Source: CAD feature listing. Evaluate the final solid. Frame: model axes, mm. Face numbers are marked on the shaded views. A direction names the side the tool comes from. Give positions to 0.01 mm unless a question says otherwise; leave off trailing zeros. Write each loop counter-clockwise with the first axis right and the second up, starting at its lowest first coordinate (ties: lowest second). Pieces come first, ordered by that corner, then holes. Notation, with made-up numbers: (8, 22) -> (55, 22) arc R21 cw to (55, 43) -> close; hole circle Ø11 at (77, -1). An arc over 180 degrees is marked (long way). Answer as a JSON object with one key per item and string values. Group by question number.
Item 1: Pull-direction query (Z, two-part tool) for the marked faces 1, 2 and 3; classes: pulls with the +Z half, pulls with the -Z half, needs draft (parallel to the pull), parting line crosses it, or undercut.
Item 2: First-contact query: pin 1 Ø7.5 at (x, y) = (92, 1) entering from -Z; pin 2 Ø7 at (x, z) = (90.5, -31) entering from +Y; pin 3 Ø4.5 at (x, y) = (-1, -5.5) entering from +Z; pin 4 Ø4 at (x, y) = (133.48, 0) entering from +Z. Flat tips, straight axial feed; report the tip coordinate or a pass-through.
Item 3: Section query A-A on y = 0. Return the cut outline in (x, z), plus the area to 3 significant figures.
Item 4: Section query C-C on z = 50. Return the cut outline in (x, y), plus the area to 3 significant figures.
Item 5: Access query for the marked faces 4, 5 and 6. Directions: +Z, -Z, +X, -X, +Y, -Y. A direction counts if a zero-diameter tool reaches every point of the face in a straight line with its end or side. Return the directions, or none.
Item 6: Ray query, probe 1 along X at (y, z) = (13.25, 50); probe 2 along Z at (x, y) = (72.5, 5); probe 3 along Y at (x, z) = (0, 0). Return the intervals inside material, ascending. Write a range as from..to.
Item 7: Section query B-B on x = 97.5. Return the cut outline in (y, z), plus the area to 3 significant figures.
Item 8: Section query D-D on y = 10. Return the cut outline in (x, z).
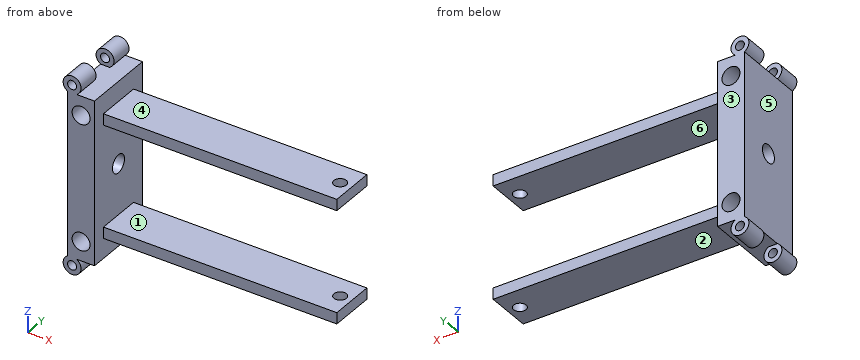
from build123d import *

# Parameters (mm, degrees)
SKETCH2_R               = 2.5
BOSS_EXTRUDE2_DEPTH     = 20
SKETCH6_W               = 9.981195927
SKETCH6_H               = 91.339745962
BOSS_EXTRUDE3_DEPTH     = 40
CUT_EXTRUDE2_DEPTH      = 69.735902352
CUT_EXTRUDE2_DEPTH_BACK = 69.735902352
SKETCH4_R               = 5
CUT_EXTRUDE1_DEPTH      = 60.368546151
CUT_EXTRUDE1_DEPTH_BACK = 60.368546151
SKETCH3_R               = 5
SKETCH3_W               = 9.330127019
SKETCH3_H               = 15
SKETCH7_W               = 6.280786139
SKETCH7_H               = 25.065781514
BOSS_EXTRUDE4_DEPTH     = 130
CUT_EXTRUDE4_DEPTH      = 165.095031026
CUT_EXTRUDE4_DEPTH_BACK = 165.095031026
SKETCH8_R               = 3.5


with BuildPart() as part:
    # Sketch2 → Boss-Extrude2 (new, symmetric)
    with BuildSketch(Plane(origin=(0, 0, 0), x_dir=(1, 0, 0), z_dir=(0, 1, 0))):
        with BuildLine():
            Line((-5, -45.669872981), (-5, 45.669872981))
            ThreePointArc((-5, 45.669872981), (-2.5, 55), (0, 45.669872981))
            Line((0, 45.669872981), (0, -45.669872981))
            ThreePointArc((0, -45.669872981), (-2.5, -55), (-5, -45.669872981))
        make_face()
        with Locations(Location((-2.5, 50, 0), (0, 0, 270))):
            Circle(SKETCH2_R, mode=Mode.SUBTRACT)
        with Locations(Location((-2.5, -50, 0), (0, 0, 270))):
            Circle(SKETCH2_R, mode=Mode.SUBTRACT)
    extrude(amount=BOSS_EXTRUDE2_DEPTH, both=True)

    # Sketch6 → Boss-Extrude3 (add)
    with BuildSketch(Plane.XZ.offset(20)):
        with Locations((4.990597963, 0)):
            Rectangle(SKETCH6_W, SKETCH6_H)
    extrude(amount=-BOSS_EXTRUDE3_DEPTH)

    # Sketch4 → Cut-Extrude2 (cut, two sides: drawn at the far end of the back side and taken through both)
    with BuildSketch(Plane(origin=(0, 20, 0), x_dir=(1, 0, 0), z_dir=(0, 1, 0)).offset(-CUT_EXTRUDE2_DEPTH_BACK)):
        with Locations(Location((2.5, 35, 0), (0, 0, 270))):
            Circle(SKETCH4_R)
        with Locations(Location((2.5, -35, 0), (0, 0, 270))):
            Circle(SKETCH4_R)
    extrude(amount=CUT_EXTRUDE2_DEPTH + CUT_EXTRUDE2_DEPTH_BACK, mode=Mode.SUBTRACT)

    # Sketch3 → Cut-Extrude1 (cut, two sides: drawn at the far end of the back side and taken through both)
    with BuildSketch(Plane(origin=(0, 0, 0), x_dir=(0, 0, -1), z_dir=(1, 0, 0)).offset(-CUT_EXTRUDE1_DEPTH_BACK)):
        Circle(SKETCH3_R)
        with Locations((50.33493649, 0)):
            Rectangle(SKETCH3_W, SKETCH3_H)
        with Locations((-50.33493649, 0)):
            Rectangle(SKETCH3_W, SKETCH3_H)
    extrude(amount=CUT_EXTRUDE1_DEPTH + CUT_EXTRUDE1_DEPTH_BACK, mode=Mode.SUBTRACT)

    # Sketch7 → Boss-Extrude4 (add)
    with BuildSketch(Plane(origin=(9.981195927, 0, 0), x_dir=(0, 0, -1), z_dir=(1, 0, 0))):
        with Locations((-31.401692569, 0)):
            Rectangle(SKETCH7_W, SKETCH7_H)
        with Locations((31.401692569, 0)):
            Rectangle(SKETCH7_W, SKETCH7_H)
    extrude(amount=BOSS_EXTRUDE4_DEPTH)

    # Sketch8 → Cut-Extrude4 (cut, two sides: drawn at the far end of the back side and taken through both)
    with BuildSketch(Plane(origin=(0, 0, 28.2612995), x_dir=(-1, 0, 0), z_dir=(0, 0, -1)).offset(-CUT_EXTRUDE4_DEPTH_BACK)):
        with Locations((-133.481195927, 0)):
            Circle(SKETCH8_R)
    extrude(amount=CUT_EXTRUDE4_DEPTH + CUT_EXTRUDE4_DEPTH_BACK, mode=Mode.SUBTRACT)


solid = part.part
Worked answers:
{
 "1": {"face 1": "undercut", "face 2": "pulls with the -Z half", "face 3": "needs draft"},
 "2": {"pin 1": "z = -34.54", "pin 2": "y = 12.53", "pin 3": "z = 54.98", "pin 4": "through"},
 "3": {"outline": "(-5, -45.67) -> (9.98, -45.67) -> (9.98, -34.54) -> (129.98, -34.54) -> (129.98, -28.26) -> (9.98, -28.26) -> (9.98, -5) -> (-5, -5) -> close; (-5, 5) -> (9.98, 5) -> (9.98, 28.26) -> (129.98, 28.26) -> (129.98, 34.54) -> (9.98, 34.54) -> (9.98, 45.67) -> (-5, 45.67) -> close; (136.98, -34.54) -> (139.98, -34.54) -> (139.98, -28.26) -> (136.98, -28.26) -> close; (136.98, 28.26) -> (139.98, 28.26) -> (139.98, 34.54) -> (136.98, 34.54) -> close; hole circle Ø10 at (2.5, -35); hole circle Ø10 at (2.5, 35)", "area": "2,610 mm^2"},
 "4": {"outline": "(-7.5, -20) -> (-5, -20) -> (-5, -7.5) -> (-7.5, -7.5) -> close; (-7.5, 7.5) -> (-5, 7.5) -> (-5, 20) -> (-7.5, 20) -> close; (0, -20) -> (2.5, -20) -> (2.5, -7.5) -> (0, -7.5) -> close; (0, 7.5) -> (2.5, 7.5) -> (2.5, 20) -> (0, 20) -> close", "area": "125 mm^2"},
 "5": {"face 4": "+Z, +X, +Y, -Y", "face 5": "-X, +Y, -Y", "face 6": "+X, +Y, -Y"},
 "6": {"probe 1": "-7.5..-5, 0..2.5", "probe 2": "-34.54..-28.26, 28.26..34.54", "probe 3": "-20..-5, 5..20"},
 "7": {"outline": "(-12.53, -34.54) -> (12.53, -34.54) -> (12.53, -28.26) -> (-12.53, -28.26) -> close; (-12.53, 28.26) -> (12.53, 28.26) -> (12.53, 34.54) -> (-12.53, 34.54) -> close", "area": "315 mm^2"},
 "8": {"outline": "(-5, -45.67) arc R5 ccw (long way) to (0, -45.67) -> (9.98, -45.67) -> (9.98, -34.54) -> (139.98, -34.54) -> (139.98, -28.26) -> (9.98, -28.26) -> (9.98, 28.26) -> (139.98, 28.26) -> (139.98, 34.54) -> (9.98, 34.54) -> (9.98, 45.67) -> (0, 45.67) arc R5 ccw (long way) to (-5, 45.67) -> close; hole circle Ø5 at (-2.5, -50); hole circle Ø5 at (-2.5, 50); hole circle Ø10 at (2.5, -35); hole circle Ø10 at (2.5, 35)"}
}
